from build123d import *

# Parameters (mm, degrees)
SKETCH1_R           = 60
SKETCH1_R_2         = 43.5
EXTRUSION1_DEPTH    = 60
EXTRUSION3_START    = -60
EXTRUSION3_DEPTH    = 60
BOSS_EXTRUDE2_START = -60
BOSS_EXTRUDE2_DEPTH = 60


with BuildPart() as part:
    # Sketch1 → Extrusion1 (new body)
    with BuildSketch(Plane.XY):
        Circle(SKETCH1_R)
        Circle(SKETCH1_R_2, mode=Mode.SUBTRACT)
    extrude(amount=EXTRUSION1_DEPTH)

    # Sketch3 → Extrusion3 (cut)
    with BuildSketch(Plane.XY.offset(60).offset(EXTRUSION3_START)):
        with BuildLine():
            Line((-0.5, 48.5), (-0.5, 43.497126342))
            ThreePointArc((-0.5, 43.497126342), (0, 43.5), (0.5, 43.497126342))
            Line((0.5, 43.497126342), (0.5, 48.5))
            Line((0.5, 48.5), (-0.5, 48.5))
        make_face()
    extrude(amount=EXTRUSION3_DEPTH, mode=Mode.SUBTRACT)

    # Sketch5 → Boss-Extrude2 (add)
    with BuildSketch(Plane.XY.offset(60).offset(BOSS_EXTRUDE2_START)):
        with BuildLine():
            Line((14.075400351, 58.325664205), (16.668444418, 68.003036408))
            Line((16.668444418, 68.003036408), (19.566221897, 67.226579273))
            Line((19.566221897, 67.226579273), (16.97317783, 57.54920707))
            ThreePointArc((16.97317783, 57.54920707), (15.529142706, 57.955549577), (14.075400351, 58.325664205))
        make_face()
        with BuildLine():
            Line((1.5, 59.981247069), (1.5, 70))
            Line((1.5, 70), (-1.5, 70))
            Line((-1.5, 70), (-1.5, 59.981247069))
            ThreePointArc((-1.5, 59.981247069), (0, 60), (1.5, 59.981247069))
        make_face()
        with BuildLine():
            Line((28.691585429, 52.695283713), (33.700961894, 61.371778265))
            Line((33.700961894, 61.371778265), (36.299038106, 59.871778265))
            Line((36.299038106, 59.871778265), (31.28966164, 51.195283713))
            ThreePointArc((31.28966164, 51.195283713), (30, 51.961524227), (28.691585429, 52.695283713))
        make_face()
        with BuildLine():
            Line((41.352486375, 43.473806719), (48.436814511, 50.558134855))
            Line((48.436814511, 50.558134855), (50.558134855, 48.436814511))
            Line((50.558134855, 48.436814511), (43.473806719, 41.352486375))
            ThreePointArc((43.473806719, 41.352486375), (42.426406871, 42.426406871), (41.352486375, 43.473806719))
        make_face()
        with BuildLine():
            Line((51.195283713, 31.28966164), (59.871778265, 36.299038106))
            Line((59.871778265, 36.299038106), (61.371778265, 33.700961894))
            Line((61.371778265, 33.700961894), (52.695283713, 28.691585429))
            ThreePointArc((52.695283713, 28.691585429), (51.961524227, 30), (51.195283713, 31.28966164))
        make_face()
        with BuildLine():
            Line((57.54920707, 16.97317783), (67.226579273, 19.566221897))
            Line((67.226579273, 19.566221897), (68.003036408, 16.668444418))
            Line((68.003036408, 16.668444418), (58.325664205, 14.075400351))
            ThreePointArc((58.325664205, 14.075400351), (57.955549577, 15.529142706), (57.54920707, 16.97317783))
        make_face()
        with BuildLine():
            Line((59.981247069, 1.5), (70, 1.5))
            Line((70, 1.5), (70, -1.5))
            Line((70, -1.5), (59.981247069, -1.5))
            ThreePointArc((59.981247069, -1.5), (60, 0), (59.981247069, 1.5))
        make_face()
        with BuildLine():
            Line((58.325664205, -14.075400351), (68.003036408, -16.668444418))
            Line((68.003036408, -16.668444418), (67.226579273, -19.566221897))
            Line((67.226579273, -19.566221897), (57.54920707, -16.97317783))
            ThreePointArc((57.54920707, -16.97317783), (57.955549577, -15.529142706), (58.325664205, -14.075400351))
        make_face()
        with BuildLine():
            Line((52.695283713, -28.691585429), (61.371778265, -33.700961894))
            Line((61.371778265, -33.700961894), (59.871778265, -36.299038106))
            Line((59.871778265, -36.299038106), (51.195283713, -31.28966164))
            ThreePointArc((51.195283713, -31.28966164), (51.961524227, -30), (52.695283713, -28.691585429))
        make_face()
        with BuildLine():
            Line((43.473806719, -41.352486375), (50.558134855, -48.436814511))
            Line((50.558134855, -48.436814511), (48.436814511, -50.558134855))
            Line((48.436814511, -50.558134855), (41.352486375, -43.473806719))
            ThreePointArc((41.352486375, -43.473806719), (42.426406871, -42.426406871), (43.473806719, -41.352486375))
        make_face()
        with BuildLine():
            Line((31.28966164, -51.195283713), (36.299038106, -59.871778265))
            Line((36.299038106, -59.871778265), (33.700961894, -61.371778265))
            Line((33.700961894, -61.371778265), (28.691585429, -52.695283713))
            ThreePointArc((28.691585429, -52.695283713), (30, -51.961524227), (31.28966164, -51.195283713))
        make_face()
        with BuildLine():
            Line((16.97317783, -57.54920707), (19.566221897, -67.226579273))
            Line((19.566221897, -67.226579273), (16.668444418, -68.003036408))
            Line((16.668444418, -68.003036408), (14.075400351, -58.325664205))
            ThreePointArc((14.075400351, -58.325664205), (15.529142706, -57.955549577), (16.97317783, -57.54920707))
        make_face()
        with BuildLine():
            Line((1.5, -59.981247069), (1.5, -70))
            Line((1.5, -70), (-1.5, -70))
            Line((-1.5, -70), (-1.5, -59.981247069))
            ThreePointArc((-1.5, -59.981247069), (0, -60), (1.5, -59.981247069))
        make_face()
        with BuildLine():
            Line((-14.075400351, -58.325664205), (-16.668444418, -68.003036408))
            Line((-16.668444418, -68.003036408), (-19.566221897, -67.226579273))
            Line((-19.566221897, -67.226579273), (-16.97317783, -57.54920707))
            ThreePointArc((-16.97317783, -57.54920707), (-15.529142706, -57.955549577), (-14.075400351, -58.325664205))
        make_face()
        with BuildLine():
            Line((-28.691585429, -52.695283713), (-33.700961894, -61.371778265))
            Line((-33.700961894, -61.371778265), (-36.299038106, -59.871778265))
            Line((-36.299038106, -59.871778265), (-31.28966164, -51.195283713))
            ThreePointArc((-31.28966164, -51.195283713), (-30, -51.961524227), (-28.691585429, -52.695283713))
        make_face()
        with BuildLine():
            Line((-41.352486375, -43.473806719), (-48.436814511, -50.558134855))
            Line((-48.436814511, -50.558134855), (-50.558134855, -48.436814511))
            Line((-50.558134855, -48.436814511), (-43.473806719, -41.352486375))
            ThreePointArc((-43.473806719, -41.352486375), (-42.426406871, -42.426406871), (-41.352486375, -43.473806719))
        make_face()
        with BuildLine():
            Line((-51.195283713, -31.28966164), (-59.871778265, -36.299038106))
            Line((-59.871778265, -36.299038106), (-61.371778265, -33.700961894))
            Line((-61.371778265, -33.700961894), (-52.695283713, -28.691585429))
            ThreePointArc((-52.695283713, -28.691585429), (-51.961524227, -30), (-51.195283713, -31.28966164))
        make_face()
        with BuildLine():
            Line((-57.54920707, -16.97317783), (-67.226579273, -19.566221897))
            Line((-67.226579273, -19.566221897), (-68.003036408, -16.668444418))
            Line((-68.003036408, -16.668444418), (-58.325664205, -14.075400351))
            ThreePointArc((-58.325664205, -14.075400351), (-57.955549577, -15.529142706), (-57.54920707, -16.97317783))
        make_face()
        with BuildLine():
            Line((-59.981247069, -1.5), (-70, -1.5))
            Line((-70, -1.5), (-70, 1.5))
            Line((-70, 1.5), (-59.981247069, 1.5))
            ThreePointArc((-59.981247069, 1.5), (-60, 0), (-59.981247069, -1.5))
        make_face()
        with BuildLine():
            Line((-58.325664205, 14.075400351), (-68.003036408, 16.668444418))
            Line((-68.003036408, 16.668444418), (-67.226579273, 19.566221897))
            Line((-67.226579273, 19.566221897), (-57.54920707, 16.97317783))
            ThreePointArc((-57.54920707, 16.97317783), (-57.955549577, 15.529142706), (-58.325664205, 14.075400351))
        make_face()
        with BuildLine():
            Line((-52.695283713, 28.691585429), (-61.371778265, 33.700961894))
            Line((-61.371778265, 33.700961894), (-59.871778265, 36.299038106))
            Line((-59.871778265, 36.299038106), (-51.195283713, 31.28966164))
            ThreePointArc((-51.195283713, 31.28966164), (-51.961524227, 30), (-52.695283713, 28.691585429))
        make_face()
        with BuildLine():
            Line((-43.473806719, 41.352486375), (-50.558134855, 48.436814511))
            Line((-50.558134855, 48.436814511), (-48.436814511, 50.558134855))
            Line((-48.436814511, 50.558134855), (-41.352486375, 43.473806719))
            ThreePointArc((-41.352486375, 43.473806719), (-42.426406871, 42.426406871), (-43.473806719, 41.352486375))
        make_face()
        with BuildLine():
            Line((-31.28966164, 51.195283713), (-36.299038106, 59.871778265))
            Line((-36.299038106, 59.871778265), (-33.700961894, 61.371778265))
            Line((-33.700961894, 61.371778265), (-28.691585429, 52.695283713))
            ThreePointArc((-28.691585429, 52.695283713), (-30, 51.961524227), (-31.28966164, 51.195283713))
        make_face()
        with BuildLine():
            Line((-16.97317783, 57.54920707), (-19.566221897, 67.226579273))
            Line((-19.566221897, 67.226579273), (-16.668444418, 68.003036408))
            Line((-16.668444418, 68.003036408), (-14.075400351, 58.325664205))
            ThreePointArc((-14.075400351, 58.325664205), (-15.529142706, 57.955549577), (-16.97317783, 57.54920707))
        make_face()
    extrude(amount=BOSS_EXTRUDE2_DEPTH)


solid = part.part
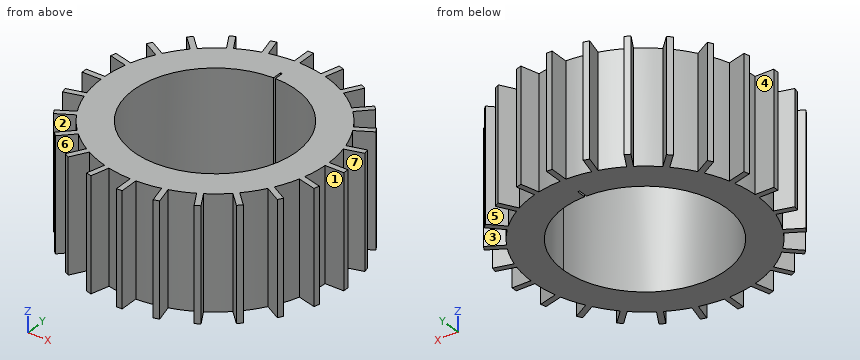
Work out the finished part from the listing and answer in its coordinate system (mm). Face numbers are marked on the shaded views. A direction names the side the tool comes from. Give positions to 0.01 mm unless a question says otherwise; leave off trailing zeros. Loops run counter-clockwise (first coordinate to the right, second up) from the corner with the lowest first, then second, coordinate; pieces in that order, holes last. Notation, with made-up numbers: (20.5, -28) - (44.5, -28) arc R9 ccw to (44.5, -14) - close; hole circle Ø6 at (-29, 22). An arc over 180 degrees is marked (long way). Answer in a Markdown table with one row per item. Add a question column.
Q1. Determine the mould class of the marked faces 5, 6 and 7 for opening direction Y: released by +Y, released by -Y, zero draft, split by the parting line, or undercut.
Q2. Each of these flat-tipped pins is pushed along its axis until it touches: P1, Ø5, axis at x = -21, z = 10, coming from the +Y side; P2, Ø1.5, axis at y = -43.5, z = 38.5, coming from the +X side; P3, Ø11, axis at x = -66.5, z = 36, coming from the +Y side; P4, Ø2, axis at x = 54, y = 31.5, coming from the -Z side. Where does it stop, or does it pass through?
Q3. The part is cut by section B-B (y = -26). Determine the outline of the cut face in (x, z), and give its area (3 significant figures).
Q4. A tool of negligible diameter and unlimited length cuts with its end or side. For the marked faces 1, 2, 3 and 4, from which of +Z, -Z, +X, -X, +Y, -Y can it reach the whole face along a straight path? Write none if from no direction.
Q5. Consider line 1 along Y through (x, z) = (0, 35); line 2 along X through (y, z) = (0, 38); line 3 along X through (y, z) = (-63, 20). Determine where each line is inside the solid, lowest interval first.
Q6. The part is cut by section A-A (x = 55). Determine the outline of the cut face in (y, z), and give its area (3 significant figures).
Q7. The part is cut by section C-C (y = 25). Determine the outline of the cut face in (x, z).
Solution:
| question | item | result |
|---|---|---|
| 1 | face 5 | released by +Y |
| 1 | face 6 | released by -Y |
| 1 | face 7 | undercut |
| 2 | P1 | stops at y = 67.51 |
| 2 | P2 | stops at x = 46.37 |
| 2 | P3 | stops at y = 34.34 |
| 2 | P4 | stops at z = 0 |
| 3 | outline | (-54.07, 0) - (-34.87, 0) - (-34.87, 60) - (-54.07, 60) - close; (34.87, 0) - (54.07, 0) - (54.07, 60) - (34.87, 60) - close |
| 3 | area | 2,300 mm² |
| 4 | face 1 | +Z, -Z, +X |
| 4 | face 2 | +Z, -Z, -Y |
| 4 | face 3 | +Z, -Z, +Y |
| 4 | face 4 | +Z, -Z, -X |
| 5 | line 1 | y = -70 to -43.5, 48.5 to 70 |
| 5 | line 2 | x = -70 to -43.5, 43.5 to 70 |
| 5 | line 3 | x = -18.43 to -15.33, -1.5 to 1.5, 15.33 to 18.43 |
| 6 | outline | (-33.49, 0) - (-30.02, 0) - (-30.02, 60) - (-33.49, 60) - close; (-23.98, 0) - (23.98, 0) - (23.98, 60) - (-23.98, 60) - close; (30.02, 0) - (33.49, 0) - (33.49, 60) - (30.02, 60) - close |
| 6 | area | 3,290 mm² |
| 7 | outline | (-54.54, 0) - (-35.6, 0) - (-35.6, 60) - (-54.54, 60) - close; (35.6, 0) - (54.54, 0) - (54.54, 60) - (35.6, 60) - close |
